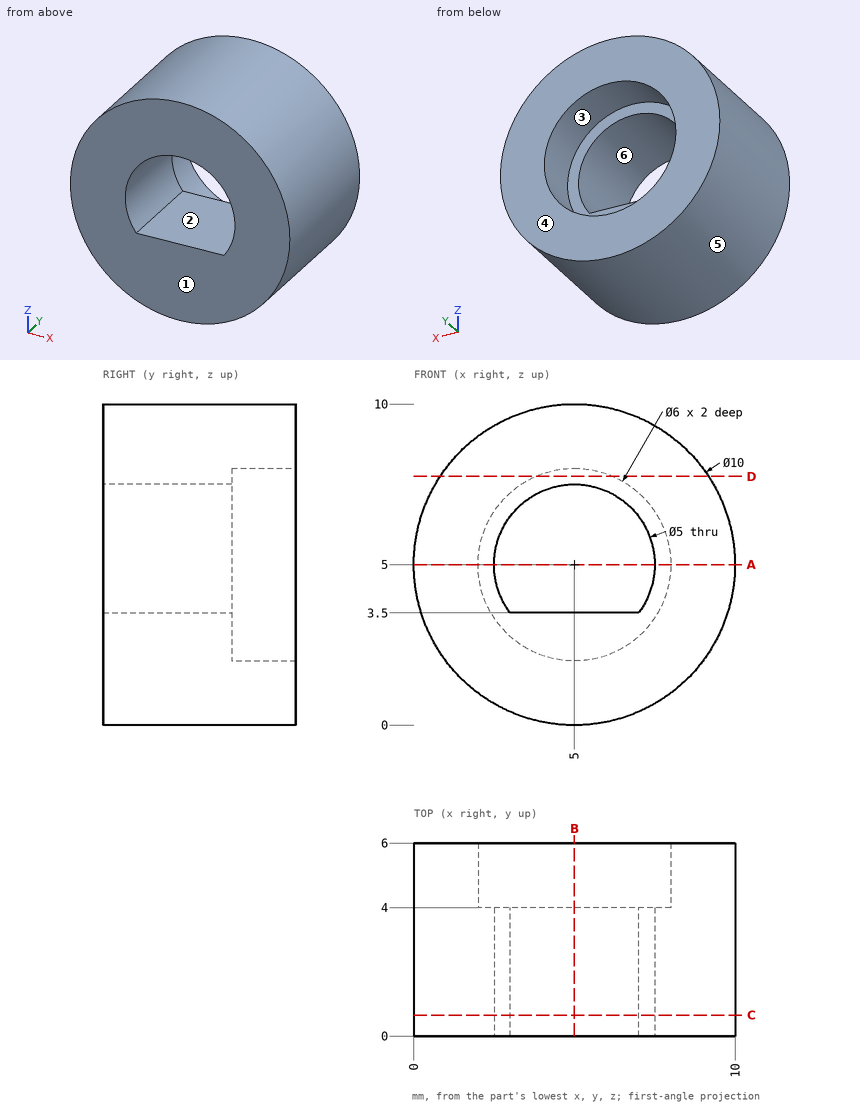
The drawing under review shows one solid part. Ordinate dimensions are in mm from its lowest x, y, z. A direction names the side the tool comes from. Give positions to 0.01 mm unless a question says otherwise; leave off trailing zeros. Order: outer loops, then holes, each group sorted by start corner. A loop starts at its lowest first (then second) coordinate and runs counter-clockwise, first axis right, second up. Notation, with made-up numbers: (-29.75, 51) - (8.25, 51) arc R37 cw to (8.25, 88) - close; hole circle Ø4 at (20.5, 0.5). An arc over 180 degrees is marked (long way). Answer as a JSON object with one key per item and string values. Group by question number.
Item 1: Take a section at B-B on x = 5. Give the boundary of the cut face in (y, z).
Item 2: Take a section at D-D on z = 7.75. Give the boundary of the cut face in (x, y), and give its area (3 significant figures).
Item 3: Take a section at C-C on y = 0.65. Give the boundary of the cut face in (x, z), and give its area (3 significant figures).
Item 4: Wall thickness on line 1 along X through (y, z) = (2.1, 5); line 2 along X through (y, z) = (4.9, 5); line 3 along Y through (x, z) = (3.25, 2.75): over which ranges is each line inside the solid? List them lowest first.
Item 5: Draft analysis for pull direction X (two halves, no side actions). For the marked faces 4, 5 and 6, state which applies: pulls with the +X half, pulls with the -X half, needs draft (parallel to the pull), parting line crosses it, or undercut.
Item 6: Machinability: for the marked faces 1, 2 and 3, which of the approach directions +Z, -Z, +X, -X, +Y, -Y give a long, thin tool a straight path to every point of the face, cutting with its end or side? Answer none if there is none.
Item 7: Take a section at A-A on z = 5. Give the boundary of the cut face in (x, y), and give its area (3 significant figures).
Item 8: Clearance check with flat-ended pins moving along their axes: pin 1 Ø1 at (y, z) = (3.5, 6) entering from +X; pin 2 Ø2 at (x, y) = (3.5, 4.5) entering from +Z; pin 3 Ø4.5 at (x, z) = (5, 5) entering from +Y. State where each tip first meets the part, or that it passes through.
Reported:
{
 "1": {"outline": "(0, 0) - (6, 0) - (6, 2) - (4, 2) - (4, 3.5) - (0, 3.5) - close; (0, 7.5) - (4, 7.5) - (4, 8) - (6, 8) - (6, 10) - (0, 10) - close"},
 "2": {"outline": "(0.82, 0) - (9.18, 0) - (9.18, 6) - (6.2, 6) - (6.2, 4) - (3.8, 4) - (3.8, 6) - (0.82, 6) - close", "area": "45.3 mm^2"},
 "3": {"outline": "circle Ø10 at (5, 5); hole (3, 3.5) - (7, 3.5) arc R2.5 ccw (long way) to start", "area": "61.7 mm^2"},
 "4": {"line 1": "0 to 2.5, 7.5 to 10", "line 2": "0 to 2, 8 to 10", "line 3": "0 to 4"},
 "5": {"face 4": "needs draft", "face 5": "parting line crosses it", "face 6": "undercut"},
 "6": {"face 1": "+Z, -Z, +X, -X, -Y", "face 2": "+Y, -Y", "face 3": "+Y"},
 "7": {"outline": "(0, 0) - (2.5, 0) - (2.5, 4) - (2, 4) - (2, 6) - (0, 6) - close; (7.5, 0) - (10, 0) - (10, 6) - (8, 6) - (8, 4) - (7.5, 4) - close", "area": "28.0 mm^2"},
 "8": {"pin 1": "x = 9.97", "pin 2": "z = 9.97", "pin 3": "y = 4"}
}
